Can you work these out from the model? Positions are in its coordinate system, mm. Face numbers are marked on the shaded views. A direction names the side the tool comes from. Give positions to 0.01 mm unless a question says otherwise; leave off trailing zeros. Loops run counter-clockwise (first coordinate to the right, second up) from the corner with the lowest first, then second, coordinate; pieces in that order, holes last. Notation, with made-up numbers: (-39.5, 36.25) - (-32.5, 36.25) arc R23 cw to (-32.5, 54.25) - close; hole circle Ø6 at (-26.5, -22.75). An arc over 180 degrees is marked (long way). Answer as a JSON object with one key per item and string values.
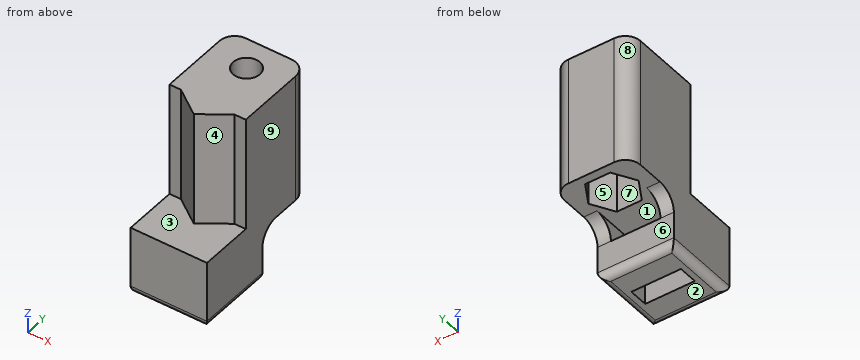
```python
from build123d import *

# Parameters (mm, degrees)
EXTRUDE_1_DEPTH     = 7
SKETCH_6_R          = 1.5
CUT_EXTRUDE_1_DEPTH = 11.934463864
CUT_EXTRUDE_2_DEPTH = 3
EXTRUDE_3_DEPTH     = 7
SKETCH_10_W         = 10
SKETCH_10_H         = 7
EXTRUDE_4_DEPTH     = 7
SKETCH_12_W         = 3.25
SKETCH_12_H         = 1.314739763
SKETCH_12_H_2       = 1.185260237
CUT_EXTRUDE_3_DEPTH = 7
CUT_EXTRUDE_4_DEPTH = 6.2
FILLET_1_R          = 2.5
FILLET_2_R          = 1
FILLET_4_R          = 2
EXTRUDE_START       = 10
SKETCH_14_R         = 1.5
EXTRUDE_5_DEPTH     = 10
SKETCH_15_W         = 10
SKETCH_15_H         = 7
EXTRUDE_6_DEPTH     = 2
CUT_EXTRUDE_5_DEPTH = 10
CUT_EXTRUDE_6_DEPTH = 10
SKETCH_19_R         = 1.75
CUT_EXTRUDE_7_DEPTH = 21.989580749


with BuildPart() as part:
    # Эскиз3 → Бобышка-Вытянуть1 (new body)
    with BuildSketch(Plane.XY):
        Polygon((0, -6.75), (-3.5, -4.25), (-5, -4.25), (-5, 4.75), (-5, 6.75), (5, 6.75), (5, -4.25), (3.5, -4.25), align=None)
    extrude(amount=EXTRUDE_1_DEPTH)

    # Эскиз6 → Вырез-Вытянуть1 (cut, through all)
    with BuildSketch(Plane(origin=(0, 0, 0), x_dir=(-1, 0, 0), z_dir=(0, 0, -1))):
        with Locations((0, 2.75)):
            Circle(SKETCH_6_R)
    extrude(amount=-CUT_EXTRUDE_1_DEPTH, mode=Mode.SUBTRACT)

    # Эскиз7 → Вырез-Вытянуть2 (cut)
    with BuildSketch(Plane(origin=(0, 0, 0), x_dir=(-1, 0, 0), z_dir=(0, 0, -1))):
        Polygon((1.58771324, 0), (3.175426481, 2.75), (1.58771324, 5.5), (-1.58771324, 5.5), (-3.175426481, 2.75), (-1.58771324, 0), align=None)
    extrude(amount=-CUT_EXTRUDE_2_DEPTH, mode=Mode.SUBTRACT)

    # Эскиз8 → Бобышка-Вытянуть3 (add)
    with BuildSketch(Plane(origin=(0, 0, 0), x_dir=(-1, 0, 0), z_dir=(0, 0, -1))):
        Polygon((-5, -1.25), (-5, -4.25), (-3.5, -4.25), (3.5, -4.25), (5, -4.25), (5, -1.25), align=None)
    extrude(amount=EXTRUDE_3_DEPTH)

    # Эскиз10 → Бобышка-Вытянуть4 (add)
    with BuildSketch(Plane.XZ.offset(4.25)):
        with Locations((0, -3.5)):
            Rectangle(SKETCH_10_W, SKETCH_10_H)
    extrude(amount=EXTRUDE_4_DEPTH)

    # Эскиз12 → Вырез-Вытянуть3 (cut)
    with BuildSketch(Plane(origin=(0, 0, -7), x_dir=(-1, 0, 0), z_dir=(0, 0, -1))):
        with Locations((-1.625, -5.592630119)):
            Rectangle(SKETCH_12_W, SKETCH_12_H)
        with Locations((1.625, -5.592630119)):
            Rectangle(SKETCH_12_W, SKETCH_12_H)
        with Locations((1.625, -6.842630119)):
            Rectangle(SKETCH_12_W, SKETCH_12_H_2)
        with Locations((-1.625, -6.842630119)):
            Rectangle(SKETCH_12_W, SKETCH_12_H_2)
    extrude(amount=-CUT_EXTRUDE_3_DEPTH, mode=Mode.SUBTRACT)

    # Эскиз13 → Вырез-Вытянуть4 (cut)
    with BuildSketch(Plane(origin=(0, -1.25, 0), x_dir=(1, 0, 0), z_dir=(0, 1, 0))):
        Polygon((0, 0), (3.25, 0), (3.25, 2.5), (-3.25, 2.5), (-3.25, 0), align=None)
    extrude(amount=-CUT_EXTRUDE_4_DEPTH, mode=Mode.SUBTRACT)

    # Скругление1
    fillet_1_edges = [part.edges().sort_by_distance(p)[0] for p in [
        (4.125, -1.25, 0),
        (-4.125, -1.25, 0),
    ]]
    fillet(fillet_1_edges, radius=FILLET_1_R)

    # Скругление2
    fillet_2_edges = [part.edges().sort_by_distance(p)[0] for p in [
        (0, -11.25, -7),
        (5, -6.25, -7),
        (-5, -6.25, -7),
        (0, -1.25, -7),
    ]]
    fillet(fillet_2_edges, radius=FILLET_2_R)

    # Скругление4
    fillet_4_edges = [part.edges().sort_by_distance(p)[0] for p in [
        (5, 6.75, 3.5),
        (-5, 6.75, 3.5),
    ]]
    fillet(fillet_4_edges, radius=FILLET_4_R)

    # Эскиз14 → Бобышка-Вытянуть5 (add)
    with BuildSketch(Plane.XY.offset(7).offset(EXTRUDE_START)):
        with BuildLine():
            Line((3.5, -4.25), (5, -4.25))
            Line((5, -4.25), (5, 4.75))
            ThreePointArc((5, 4.75), (4.414213562, 6.164213562), (3, 6.75))
            Line((3, 6.75), (-3, 6.75))
            ThreePointArc((-3, 6.75), (-4.414213562, 6.164213562), (-5, 4.75))
            Line((-5, 4.75), (-5, -4.25))
            Line((-5, -4.25), (-3.5, -4.25))
            Line((-3.5, -4.25), (0, -6.75))
            Line((0, -6.75), (3.5, -4.25))
        make_face()
        with Locations(Location((0, 2.75, 0), (0, 0, 180))):
            Circle(SKETCH_14_R, mode=Mode.SUBTRACT)
    extrude(amount=-EXTRUDE_5_DEPTH)

    # Эскиз15 → Бобышка-Вытянуть6 (add)
    with BuildSketch(Plane.XY):
        with Locations((0, -7.75)):
            Rectangle(SKETCH_15_W, SKETCH_15_H)
    extrude(amount=EXTRUDE_6_DEPTH)

    # Эскиз17 → Вырез-Вытянуть5 (cut)
    with BuildSketch(Plane(origin=(0, 0, 0), x_dir=(-1, 0, 0), z_dir=(0, 0, -1))):
        Polygon((1.58771324, 0), (3.175426481, 2.75), (1.58771324, 5.5), (-1.58771324, 5.5), (-3.175426481, 2.75), (-1.58771324, 0), align=None)
    extrude(amount=-CUT_EXTRUDE_5_DEPTH, mode=Mode.SUBTRACT)

    # Эскиз18 → Вырез-Вытянуть6 (cut)
    with BuildSketch(Plane(origin=(0, 0, 0), x_dir=(-1, 0, 0), z_dir=(0, 0, -1))):
        Polygon((1.645448267, -0.1), (3.290896534, 2.75), (1.645448267, 5.6), (-1.645448267, 5.6), (-3.290896534, 2.75), (-1.645448267, -0.1), align=None)
    extrude(amount=-CUT_EXTRUDE_6_DEPTH, mode=Mode.SUBTRACT)

    # Эскиз19 → Вырез-Вытянуть7 (cut, through all)
    with BuildSketch(Plane(origin=(0, 0, 10), x_dir=(-1, 0, 0), z_dir=(0, 0, -1))):
        with Locations((0, 2.75)):
            Circle(SKETCH_19_R)
    extrude(amount=-CUT_EXTRUDE_7_DEPTH, mode=Mode.SUBTRACT)


solid = part.part
```
1) Which directions (+Z, -Z, +X, -X, +Y, -Y) give clear straight access to the entire face, cutting with the end or side of a thin tool? Please do the marked faces 1, 2, 3, 4 and 5.
Check sheet entries:
{"face 1": "+Y", "face 2": "-Z, +X, -X, +Y, -Y", "face 3": "+Z, -Y", "face 4": "+Z, +X, -Y", "face 5": "-Z"}
2) Imagine slicing it at B-B on y = -8.5. Write out the boundary of the cut face in (x, z), and give its area (3 significant figures).
Check sheet entries:
{"outline": "(-5, -6) arc R1 ccw to (-4, -7) - (4, -7) arc R1 ccw to (5, -6) - (5, 2) - (-5, 2) - close", "area": "89.6 mm2"}
3) Imagine slicing it at A-A on z = 11.5. Write out the boundary of the cut face in (x, y).
Check sheet entries:
{"outline": "(-5, -4.25) - (-3.5, -4.25) - (0, -6.75) - (3.5, -4.25) - (5, -4.25) - (5, 4.75) arc R2 ccw to (3, 6.75) - (-3, 6.75) arc R2 ccw to (-5, 4.75) - close; hole circle Ø3.5 at (0, 2.75)"}
4) Imagine slicing it at C-C on x = 1.25. Give the number of separate pieces and of enclosed holes in the cut face, and give its area (3 significant figures).
Check sheet entries:
{"separate pieces": "3", "enclosed holes": "0", "area": "194 mm2"}
5) Imagine slicing it at D-D on z = 8.5. Write out the boundary of the cut face in (x, y).
Check sheet entries:
{"outline": "(-5, -4.25) - (-3.5, -4.25) - (0, -6.75) - (3.5, -4.25) - (5, -4.25) - (5, 4.75) arc R2 ccw to (3, 6.75) - (-3, 6.75) arc R2 ccw to (-5, 4.75) - close; hole (-3.29, 2.75) - (-1.65, -0.1) - (1.65, -0.1) - (3.29, 2.75) - (1.65, 5.6) - (-1.65, 5.6) - close"}
6) I need wall thicknesses on L1, parallel to Y at x = -1, z = -4.25; L2, parallel to Z at x = 0.75, y = 0.5; L3, parallel to Z at x = 2, y = -4.25. Which ranges of each line are inside material? Lowest first, please.
Check sheet entries:
{"L1": "-11.25 to -7.44, -4.94 to -1.25", "L2": "10 to 17", "L3": "-7 to -2.5, 0 to 17"}
7) If we mould it in two halves opening along X, with no side actions, what happens to the marked faces 6, 7, 8 and 9? For each: released by +X, released by -X, zero draft, split by the parting line, or undercut.
Check sheet entries:
{"face 6": "zero draft", "face 7": "undercut", "face 8": "released by -X", "face 9": "released by +X"}
8) I'm going to push flat-ended pins straight in: P1, Ø1.7, axis at x = -1, y = 2, coming from the -Z side; P2, Ø2, axis at x = -0.5, z = -5, coming from the +Y side; P3, Ø2, axis at x = 0, y = 2.75, coming from the -Z side; P4, Ø1.2, axis at x = 1, z = -1, coming from the +Y side. Where does each tip first touch, or does it pass through?
Check sheet entries:
{"P1": "z = 10", "P2": "y = -1.25", "P3": "through", "P4": "y = -7.45"}
